Check sheet for the modelled part. Datum: model origin and axes. Units: mm. A direction names the side the tool comes from. Give positions to 0.01 mm unless a question says otherwise; leave off trailing zeros. Loops run counter-clockwise (first coordinate to the right, second up) from the corner with the lowest first, then second, coordinate; pieces in that order, holes last. Notation, with made-up numbers: (-29, 13.25) - (8, 13.25) arc R22 ccw to (8, 27.25) - close; hole circle Ø11 at (-5.75, -33.75). An arc over 180 degrees is marked (long way). Use CSV: the item, a comma, the result in double quotes.
from build123d import *

# Parameters (mm, degrees)
SKETCH1_W                                         = 199
SKETCH1_H                                         = 199
BOSS_EXTRUDE1_DEPTH                               = 5
SKETCH2_W                                         = 5
SKETCH2_H                                         = 25
BOSS_EXTRUDE2_DEPTH                               = 18.8
SKETCH3_W                                         = 5
SKETCH3_H                                         = 25
BOSS_EXTRUDE3_DEPTH                               = 46.4
SKETCH4_W                                         = 5
SKETCH4_H                                         = 25
BOSS_EXTRUDE4_DEPTH                               = 91.8
SKETCH5_W                                         = 5
SKETCH5_H                                         = 25
BOSS_EXTRUDE5_DEPTH                               = 157
SKETCH6_R                                         = 4.5
CUT_EXTRUDE1_DEPTH                                = 325.724498614
SKETCH12_W                                        = 6
SKETCH12_H                                        = 42
CUT_EXTRUDE3_DEPTH                                = 5
M3X0_5_TAPPED_HOLE1_D                             = 2.5
M3X0_5_TAPPED_HOLE1_DEPTH                         = 4
M3X0_5_TAPPED_HOLE1_TIP                           = 0.751075774
CSK_FOR_M2_5_FLAT_HEAD_MACHINE_SCREW1_D           = 2.9
CSK_FOR_M2_5_FLAT_HEAD_MACHINE_SCREW1_DEPTH       = 5
CSK_FOR_M2_5_FLAT_HEAD_MACHINE_SCREW1_CSINK_D     = 5.5
CSK_FOR_M2_5_FLAT_HEAD_MACHINE_SCREW1_CSINK_ANGLE = 90
M2_5X0_45_TAPPED_HOLE1_D                          = 2.05
M2_5X0_45_TAPPED_HOLE1_DEPTH                      = 4
M2_5X0_45_TAPPED_HOLE1_CSINK_D                    = 2.55
M2_5X0_45_TAPPED_HOLE1_CSINK_ANGLE                = 90
M2_5X0_45_TAPPED_HOLE1_TIP                        = 0.615882135
M3X0_5_TAPPED_HOLE2_D                             = 2.5
M3X0_5_TAPPED_HOLE2_DEPTH                         = 4.3
M3X0_5_TAPPED_HOLE2_CSINK_D                       = 3.05
M3X0_5_TAPPED_HOLE2_CSINK_ANGLE                   = 90
M3X0_5_TAPPED_HOLE2_TIP                           = 0.751075774


with BuildPart() as part:
    # Sketch1 → Boss-Extrude1 (new body)
    with BuildSketch(Plane(origin=(0, 0, 0), x_dir=(1, 0, 0), z_dir=(0, 1, 0))):
        with Locations((99.5, -99.5)):
            Rectangle(SKETCH1_W, SKETCH1_H)
    extrude(amount=BOSS_EXTRUDE1_DEPTH)

    # Sketch2 → Boss-Extrude2 (add)
    with BuildSketch(Plane(origin=(0, 5, 0), x_dir=(1, 0, 0), z_dir=(0, 1, 0))):
        with Locations((2.5, -63)):
            Rectangle(SKETCH2_W, SKETCH2_H)
    extrude(amount=BOSS_EXTRUDE2_DEPTH)

    # Sketch3 → Boss-Extrude3 (add)
    with BuildSketch(Plane(origin=(0, 23.8, 0), x_dir=(1, 0, 0), z_dir=(0, 1, 0))):
        with Locations((2.5, -63)):
            Rectangle(SKETCH3_W, SKETCH3_H)
    extrude(amount=BOSS_EXTRUDE3_DEPTH)

    # Sketch4 → Boss-Extrude4 (add)
    with BuildSketch(Plane(origin=(0, 70.2, 0), x_dir=(1, 0, 0), z_dir=(0, 1, 0))):
        with Locations((2.5, -63)):
            Rectangle(SKETCH4_W, SKETCH4_H)
    extrude(amount=BOSS_EXTRUDE4_DEPTH)

    # Sketch5 → Boss-Extrude5 (add)
    with BuildSketch(Plane(origin=(0, 5, 0), x_dir=(1, 0, 0), z_dir=(0, 1, 0))):
        with Locations((196.5, -63)):
            Rectangle(SKETCH5_W, SKETCH5_H)
    extrude(amount=BOSS_EXTRUDE5_DEPTH)

    # Sketch6 → Cut-Extrude1 (cut, through all)
    with BuildSketch(Plane.ZY):
        with Locations((63, 149.5)):
            Circle(SKETCH6_R)
    extrude(amount=-CUT_EXTRUDE1_DEPTH, mode=Mode.SUBTRACT)

    # Sketch12 → Cut-Extrude3 (cut)
    with BuildSketch(Plane(origin=(0, 5, 0), x_dir=(1, 0, 0), z_dir=(0, 1, 0))):
        with Locations((10, -116.5)):
            Rectangle(SKETCH12_W, SKETCH12_H)
    extrude(amount=-CUT_EXTRUDE3_DEPTH, mode=Mode.SUBTRACT)

    # M3x0.5 Tapped Hole1
    with Locations(Plane(origin=(0, 5, 0), x_dir=(1, 0, 0), z_dir=(0, 1, 0))):
        with Locations((34, -97.8), (44.31875, -120)):
            Hole(M3X0_5_TAPPED_HOLE1_D / 2, depth=M3X0_5_TAPPED_HOLE1_DEPTH)
            with Locations((0, 0, -(M3X0_5_TAPPED_HOLE1_DEPTH + M3X0_5_TAPPED_HOLE1_TIP / 2))):  # 118° drill point
                Cone(0, M3X0_5_TAPPED_HOLE1_D / 2, M3X0_5_TAPPED_HOLE1_TIP, mode=Mode.SUBTRACT)

    # CSK for M2.5 Flat Head Machine Screw1
    with Locations(Plane(origin=(5, 62, 65.5), x_dir=(0, 0, 1), z_dir=(1, 0, 0))):
        with Locations((0, 0), (0, 10), (0, 20), (0, 30)):
            CounterSinkHole(CSK_FOR_M2_5_FLAT_HEAD_MACHINE_SCREW1_D / 2, CSK_FOR_M2_5_FLAT_HEAD_MACHINE_SCREW1_CSINK_D / 2, depth=CSK_FOR_M2_5_FLAT_HEAD_MACHINE_SCREW1_DEPTH, counter_sink_angle=CSK_FOR_M2_5_FLAT_HEAD_MACHINE_SCREW1_CSINK_ANGLE)

    # M2.5x0.45 Tapped Hole1
    with Locations(Plane(origin=(0, 5, 0), x_dir=(1, 0, 0), z_dir=(0, 1, 0))):
        with Locations((132.323297508, -175.500631971), (132.323297508, -158.999368029), (176.776702492, -158.999368029), (176.776702492, -175.500631971)):
            CounterSinkHole(M2_5X0_45_TAPPED_HOLE1_D / 2, M2_5X0_45_TAPPED_HOLE1_CSINK_D / 2, depth=M2_5X0_45_TAPPED_HOLE1_DEPTH, counter_sink_angle=M2_5X0_45_TAPPED_HOLE1_CSINK_ANGLE)
            with Locations((0, 0, -(M2_5X0_45_TAPPED_HOLE1_DEPTH + M2_5X0_45_TAPPED_HOLE1_TIP / 2))):  # 118° drill point
                Cone(0, M2_5X0_45_TAPPED_HOLE1_D / 2, M2_5X0_45_TAPPED_HOLE1_TIP, mode=Mode.SUBTRACT)

    # M3x0.5 Tapped Hole2
    with Locations(Plane(origin=(0, 5, 0), x_dir=(1, 0, 0), z_dir=(0, 1, 0))):
        with Locations((167.156, -81.28)):
            CounterSinkHole(M3X0_5_TAPPED_HOLE2_D / 2, M3X0_5_TAPPED_HOLE2_CSINK_D / 2, depth=M3X0_5_TAPPED_HOLE2_DEPTH, counter_sink_angle=M3X0_5_TAPPED_HOLE2_CSINK_ANGLE)
            with Locations((0, 0, -(M3X0_5_TAPPED_HOLE2_DEPTH + M3X0_5_TAPPED_HOLE2_TIP / 2))):  # 118° drill point
                Cone(0, M3X0_5_TAPPED_HOLE2_D / 2, M3X0_5_TAPPED_HOLE2_TIP, mode=Mode.SUBTRACT)


solid = part.part
1. Go/stop test with flat-tipped pins: pin 1 Ø2.5 at (y, z) = (32, 65.5) entering from -X; pin 2 Ø2 at (x, z) = (101.5, 67) entering from +Y; pin 3 Ø1.5 at (x, z) = (167.156, 81.28) entering from +Y. Record where each tip stops, or that it passes through.
Completed:
pin 1,"stops at x = 194"
pin 2,"stops at y = 5"
pin 3,"stops at y = 0.4"
2. Scan lines: line 1 along X through (y, z) = (4.2, 120); line 2 along Y through (x, z) = (1.9, 65.5); line 3 along X through (y, z) = (122.5, 59). Record each from-to range of solid material in increasing order.
Completed:
line 1,"x = 0 to 7, 13 to 43.07, 45.57 to 199"
line 2,"y = 0 to 30.55, 33.45 to 40.55, 43.45 to 50.55, 53.45 to 60.55, 63.45 to 145.76, 153.24 to 162"
line 3,"x = 0 to 5, 194 to 199"
3. Release check for a two-part mould opening along Y. For faces 4 (the face through (10, 3, 95.5)), 5 (the face through (2, 162, 63)), 6 (the face through (196.46, 145.11, 62.02)), 7 (the face through (2.46, 145.11, 62.02)) record: released by +Y, released by -Y, zero draft, split by the parting line, or undercut.
Completed:
face 4,"zero draft"
face 5,"released by +Y"
face 6,"undercut"
face 7,"undercut"
4. Sectioned sample at B-B, the plane y = 149.5. Record the boundary of the cut face in (x, z).
Completed:
outline,"(0, 50.5) - (5, 50.5) - (5, 58.5) - (0, 58.5) - close; (0, 67.5) - (5, 67.5) - (5, 75.5) - (0, 75.5) - close; (194, 50.5) - (199, 50.5) - (199, 58.5) - (194, 58.5) - close; (194, 67.5) - (199, 67.5) - (199, 75.5) - (194, 75.5) - close"
5. Sectioned sample at C-C, the plane x = 120. Record the boundary of the cut face in (y, z), and give its area (3 significant figures).
Completed:
outline,"(0, 0) - (5, 0) - (5, 199) - (0, 199) - close"
area,"995 mm²"
6. Set-up check for faces 1 (the face through (2, 82, 50.5)), 2 (the face through (194, 82, 63)), 3 (the face through (7, 3, 117)): record each of +Z, -Z, +X, -X, +Y, -Y from which the full face is reachable in a straight line by a thin tool's end or side.
Completed:
face 1,"-Z, +X, -X, +Y"
face 2,"+Z, -Z, +Y"
face 3,"+Y, -Y"
7. Sectioned sample at A-A, the plane y = 92. Record the boundary of the cut face in (x, z).
Completed:
outline,"(0, 50.5) - (5, 50.5) - (5, 75.5) - (0, 75.5) - close; (194, 50.5) - (199, 50.5) - (199, 75.5) - (194, 75.5) - close"
